Here's how the part is built. I have some questions about the finished solid (model axes, mm). A direction names the side the tool comes from. Give positions to 0.01 mm unless a question says otherwise; leave off trailing zeros. Write each loop counter-clockwise with the first axis right and the second up, starting at its lowest first coordinate (ties: lowest second). Pieces come first, ordered by that corner, then holes. Notation, with made-up numbers: (15, 28.5) - (31, 28.5) arc R15 ccw to (31, 48.5) - close; hole circle Ø4 at (20.25, 21.25). An arc over 180 degrees is marked (long way). Use a Markdown table: item, result.
Autodesk Fusion 360 part; units mm, degrees
sketch "Sketch1" plane through (0, 0, 0) normal (0, 1, 0) x (1, 0, 0)
  circle A0 centre (0, 0) radius 13.25
  dimension "d1" = 26.5
extrude "Extrude1" add sketch "Sketch1" along normal blind 15 makes body 1
sketch "Sketch2" plane through (0, 0, 0) normal (0, 0, 1) x (1, 0, 0)
  circle A0 centre (0.132, 10.5) radius 2.35
  dimension "d5" = 4.7
  dimension "d10" = 10.5
extrude "Extrude2" add sketch "Sketch2" along normal blind 15 bodies 1
sketch "Sketch3" plane through (0, 0, 0) normal (0, 1, 0) x (1, 0, 0)
  circle A0 centre (0, 0) radius 12.5
  dimension "d8" = 25
extrude "Extrude3" cut sketch "Sketch3" along normal through all bodies 1
sketch "Sketch4" plane through (0, 0, 0) normal (0, 1, 0) x (1, 0, 0)
  line L0 (-16, -39.1044) -> (19, -39.1044)
  line L1 (19, 20.8956) -> (-16, 20.8956)
  line L2 (-16, 20.8956) -> (-16, -39.1044)
  line L3 (15.75, -2.5252) -> (10.75, -2.5252)
  line L4 (10.75, -2.5252) -> (10.75, 2.4748)
  line L5 (10.75, 2.4748) -> (15.75, 2.4748)
  line L6 (15.75, 2.4748) -> (15.75, -2.5252)
  line L7 (15.75, -2.5252) -> (10.75, 2.4748) construction
  line L8 (10.75, -2.5252) -> (15.75, 2.4748) construction
  circle A0 centre (0, 0) radius 13.25
  line L9 (19, 20.8956) -> (19, -39.1044)
  line L10 (32, -21) -> (64.7832, -21) construction
  line L11 (64.7832, -21) -> (64.7832, -31) construction
  line L12 (64.7832, -31) -> (32, -31) construction
  line L13 (32, -31) -> (32, -21) construction
  line L14 (0, -45) -> (0, 21) construction
  circle A1 centre (-5, 15) radius 1
  circle A2 centre (5, 15) radius 1
  line L15 (-19, 0) -> (28, 0) construction
  circle A3 centre (-5, -34) radius 1
  circle A4 centre (5, -34) radius 1
  line L16 (-10, -29) -> (10, -29)
  line L17 (10, -29) -> (10, 10)
  line L18 (10, 10) -> (-10, 10)
  line L19 (-10, 10) -> (-10, -29)
  circle A5 centre (0, 0) radius 5
  line L20 (-1.9268, -29) -> (2, -29)
  line L21 (2, -29) -> (2, -35)
  line L22 (2, -35) -> (-1.9268, -35)
  line L23 (-1.9268, -35) -> (-1.9268, -29)
  line L24 (-1.9609, 10) -> (2, 10)
  line L25 (2, 10) -> (2, 16)
  line L26 (2, 16) -> (-1.9609, 16)
  line L27 (-1.9609, 16) -> (-1.9609, 10)
  dimension "d13" = 5
  dimension "d14" = 5
  dimension "d15" = 2
  dimension "d16" = 49
  dimension "d23" = 35
  dimension "d24" = 60
  dimension "d25" = 39
  dimension "d26" = 20
  dimension "d27" = 10
  dimension "d28" = 10
  dimension "d29" = 10
extrude "Extrude11" add sketch "Sketch4" against normal blind 7 separate body contours L0 L1 L2 L9 | L3 L4 L5 A0 L17 | A0 L19 | A0 L17 L18 | A0 L18 L19 | A0 L18 L25 | A0 L18 L27 makes body 2
extrude "Extrude10" add sketch "Sketch4" against normal blind 1 contours L0 L1 L2 L9 | L3 L4 L5 A0 L17 | A0 L16 L17 L19 L20 | A0 L17 L18 L19 L24 | A0 L19 | A0 L17 L18 | A0 L18 L19 | L16 L20 L21 L22 L23 | A0 L18 L25 | A0 L18 L27 | A0 L18 L24 L25 L27 | A0 L25 L26 L27 bodies 2 1
extrude "Extrude12" cut sketch "Sketch4" along normal blind 13 contours L3 L5 L6 A0 | L3 L4 L5 A0 bodies 2
chamfer "Chamfer1" distance 3 angle 45 4 edges at (-16, -7, 9.1044) (1.5, -7, 39.1044) (19, -7, 9.1044) (1.5, -7, -20.8956) on bodies 2
chamfer "Chamfer2" distance 1 angle 45 4 edges at (19, 0, 9.1044) (1.5, 0, 39.1044) (-16, 0, 9.1044) (1.5, 0, -20.8956) on bodies 2
Item 1: Will these pins go through, and if not, where does the flat tip stop? pin 1 Ø16 at (x, z) = (0, 0) entering from -Y; pin 2 Ø5 at (x, y) = (-6.5, 8.5) entering from +Z; pin 3 Ø2 at (x, z) = (5, 18) entering from +Y.
Values:
| item | result |
|---|---|
| pin 1 | stops at y = -1 |
| pin 2 | stops at z = 12.63 |
| pin 3 | stops at y = 0 |
Item 2: If we section it at B-B, the plane x = 15: Write out the boundary of the cut face in (y, z).
Values:
| item | result |
|---|---|
| outline | (-7, -17.9) - (-4, -20.9) - (-1, -20.9) - (0, -19.9) - (0, -2.47) - (-7, -2.47) - close; (-7, 2.53) - (0, 2.53) - (0, 38.1) - (-1, 39.1) - (-4, 39.1) - (-7, 36.1) - close |
Item 3: I need wall thicknesses on line 1 along Z through (x, y) = (5, -3); line 2 along X through (y, z) = (-2, -15); line 3 along Z through (x, y) = (0, 7.5). Which ranges of each line are inside material? Lowest first, please. Write a range as [from, to].
Values:
| item | result |
|---|---|
| line 1 | z = [-20.9, -16], [-14, -10], [29, 33], [35, 39.1] |
| line 2 | x = [-16, -6], [-4, -1.96], [2, 4], [6, 19] |
| line 3 | z = [-13.25, -12.5], [12.5, 13.25] |
Item 4: If we section it at D-D, the plane z = 14: Write out the boundary of the cut face in (x, y).
Values:
| item | result |
|---|---|
| outline | (-16, -4) - (-13, -7) - (-10, -7) - (-10, -1) - (10, -1) - (10, -7) - (16, -7) - (19, -4) - (19, -1) - (18, 0) - (-15, 0) - (-16, -1) - close; circle Ø4.7 at (0.13, 10.5) |
Item 5: Thinking about a two-plate mould opening in X: for faces 1 (the flat face through (0, 11, 15)), 2 (the flat face through (-6, -4, 29)), 3 (the flat face through (-14, -6, 9)), which applies, +X half, -X half, draft (parallel to the pull), parting line (faces both ways), or undercut?
Values:
| item | result |
|---|---|
| face 1 | draft |
| face 2 | undercut |
| face 3 | -X half |
Item 6: If we section it at C-C, the plane z = 34: Write out the boundary of the cut face in (x, y).
Values:
| item | result |
|---|---|
| outline | (-16, -4) - (-13, -7) - (-6, -7) - (-6, 0) - (-15, 0) - (-16, -1) - close; (-4, -7) - (-1.93, -7) - (-1.93, -1) - (2, -1) - (2, -7) - (4, -7) - (4, 0) - (-4, 0) - close; (6, -7) - (16, -7) - (19, -4) - (19, -1) - (18, 0) - (6, 0) - close |
Item 7: If we section it at A-A, the plane z = 0: Write out the boundary of the cut face in (x, y), plus the area to 4 significant figures.
Values:
| item | result |
|---|---|
| outline | (-16, -4) - (-13, -7) - (-10, -7) - (-10, -1) - (-5, -1) - (-5, 0) - (-12.5, 0) - (-12.5, 15) - (-13.25, 15) - (-13.25, 0) - (-15, 0) - (-16, -1) - close; (5, -1) - (10, -1) - (10, -7) - (10.75, -7) - (10.75, 0) - (5, 0) - close; (12.5, 13) - (13.25, 13) - (13.25, 15) - (12.5, 15) - close; (15.75, -7) - (16, -7) - (19, -4) - (19, -1) - (18, 0) - (15.75, 0) - close |
| area | 82.75 mm2 |
Item 8: For faces 4 (the flat face through (11, -7, 9)), 5 (the flat face through (10.75, -3, 0)), 6 (the flat face through (10, -4, 10)), 7 (the flat face through (-16, -2, 9)), 8 (the cylindrical face through (11.923, 7.395, 3.755)), which set-ups out of +Z, -Z, +X, -X, +Y, -Y let a thin tool reach every point of the face, with its end or its side?
Values:
| item | result |
|---|---|
| face 4 | +Z, -Z, +X, -X, -Y |
| face 5 | +Y, -Y |
| face 6 | -Y |
| face 7 | +Z, -Z, -X, +Y, -Y |
| face 8 | +Y |
